Part print with two shaded views. Sizes in mm from the minimum x, y, z corner. A direction names the side the tool comes from. Give positions to 0.01 mm unless a question says otherwise; leave off trailing zeros. Write each loop counter-clockwise with the first axis right and the second up, starting at its lowest first coordinate (ties: lowest second). Pieces come first, ordered by that corner, then holes.
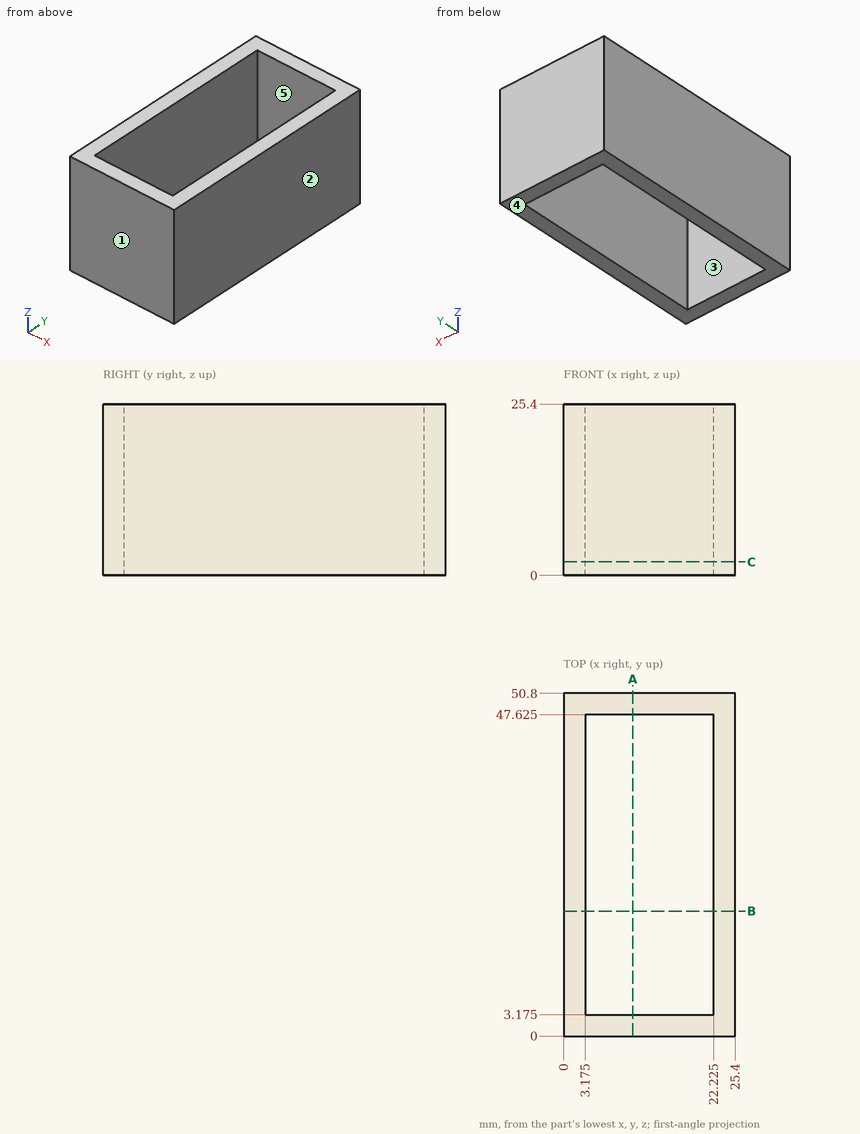
1) Saw through at B-B, the plane y = 18.5. Write the cut outline in (x, z) (3 decimals), then the cut area to 3 significant figures.
Answers follow:
outline: (0, 0) - (3.175, 0) - (3.175, 25.4) - (0, 25.4) - close; (22.225, 0) - (25.4, 0) - (25.4, 25.4) - (22.225, 25.4) - close
area: 161 mm2
2) 3-axis set-ups, long thin cutter, end or side, ignore diameter. For the marked faces 4 and 5: which of +Z, -Z, +X, -X, +Y, -Y reach the whole face in a straight line?
Answers follow:
face 4: -Z, +X, -X, +Y, -Y
face 5: +Z, -Z
3) Pin check, flat tips, straight feed: pin 1 Ø12 at (y, z) = (5.5, 9.5) entering from -X; pin 2 Ø8 at (x, y) = (8, 14.5) entering from +Z. Stop position of each tip, or through.
Answers follow:
pin 1: stops at x = 0
pin 2: passes through
4) Saw through at A-A, the plane x = 10.25. Write the cut outline in (y, z) (3 decimals).
Answers follow:
outline: (0, 0) - (3.175, 0) - (3.175, 25.4) - (0, 25.4) - close; (47.625, 0) - (50.8, 0) - (50.8, 25.4) - (47.625, 25.4) - close
5) Wall check: L1, parallel to Y at x = 10, z = 9.25 (3 decimals); L2, parallel to X at y = 8, z = 15.25 (3 decimals). Give the ranges that are in metal, low to high.
Answers follow:
L1: y = 0 to 3.175, 47.625 to 50.8
L2: x = 0 to 3.175, 22.225 to 25.4
6) Saw through at C-C, the plane z = 2. Write the cut outline in (x, y) (3 decimals), then the cut area to 3 significant figures.
Answers follow:
outline: (0, 0) - (25.4, 0) - (25.4, 50.8) - (0, 50.8) - close; hole (3.175, 3.175) - (22.225, 3.175) - (22.225, 47.625) - (3.175, 47.625) - close
area: 444 mm2
7) Two-plate mould, pull along X, no slides. Class the marked faces 1, 2 and 3: +X half, -X half, draft (parallel to the pull), parting line (faces both ways), or undercut.
Answers follow:
face 1: draft
face 2: +X half
face 3: undercut
